Read the model definition and answer for the solid it produces. Units are mm, in the model's axes. A direction names the side the tool comes from. Give positions to 0.01 mm unless a question says otherwise; leave off trailing zeros. Order: outer loops, then holes, each group sorted by start corner. A loop starts at its lowest first (then second) coordinate and runs counter-clockwise, first axis right, second up.
Solid Edge part; units mm, degrees
sketch "Sketch1" plane through (0, 0, 0) normal (0, 0, 1) x (1, 0, 0)
  line L0 (0, -15) -> (120, -15)
  line L1 (0, 15) -> (120, 15)
  arc A0 (120, 15) -> (120, -15) centre (120, 0) cw
  arc A1 (0, -15) -> (0, 15) centre (0, 0) cw
extrude "Protrusion1" add sketch "Sketch1" against normal blind 6
sketch "Sketch2" plane through (0, 0, 0) normal (0, 0, 1) x (1, 0, 0)
  circle A0 centre (0, 0) radius 8
  circle A1 centre (120, 0) radius 8
extrude "VaciadoExtruido_1" cut sketch "Sketch2" against normal blind 5
sketch "Sketch3" plane through (0, 0, -5) normal (0, 0, 1) x (1, 0, 0)
  circle A0 centre (0, 0) radius 4.5
  circle A1 centre (120, 0) radius 4.5
extrude "Cutout1" cut sketch "Sketch3" against normal through all
chamfer "Chaflán_1" distance 3 angle 45 4 edges at (60, -15, -6) (135, 0, -6) (60, 15, -6) (-15, 0, -6)
1) For a pull along Y with two mould halves and no side action, classify faces 3 (the face through (135, 0, -1)), 4 (the face through (123.4, -3.4, -5)), 5 (the face through (59, -13, -5)) as released by +Y, released by -Y, zero draft, split by the parting line, or undercut.
Final values:
face 3: split by the parting line
face 4: undercut
face 5: released by -Y
2) Given pin 1 (5 mm diameter, centred on x = 124, y = 3, fed in from +Z); pin 2 (1 mm diameter, centred on x = 104, z = -4, fed in from +Y); pin 3 (1 mm diameter, centred on x = 105.5, z = -5, fed in from +Y), each flat-ended and moving along its own axis, determine where each tip first touches the part or whether it passes through.
Final values:
pin 1: stops at z = -5
pin 2: stops at y = 14.5
pin 3: stops at y = 13.5
3) A tool of negligible diameter and unlimited length cuts with its end or side. For faces 1 (the face through (127.63, 2.4, -2.46)), 2 (the face through (-0.59, 4.46, -5.49)), from which of +Z, -Z, +X, -X, +Y, -Y can it reach the whole face along a straight path? Write none if from no direction.
Final values:
face 1: +Z
face 2: +Z, -Z
4) Consider L1, parallel to X at y = -6.5, z = -0.6; L2, parallel to X at y = 0.75, z = -1.85; L3, parallel to Y at x = 120, z = -1.35. Determine where each line is inside the solid, lowest interval first.
Final values:
L1: x = -13.52 to -4.66, 4.66 to 115.34, 124.66 to 133.52
L2: x = -14.98 to -7.96, 7.96 to 112.04, 127.96 to 134.98
L3: y = -15 to -8, 8 to 15
5) The part is cut by section A-A on y = 0. Determine the outline of the cut face in (x, z), and give its area (3 significant figures).
Final values:
outline: (-15, -3) - (-12, -6) - (-4.5, -6) - (-4.5, -5) - (-8, -5) - (-8, 0) - (-15, 0) - close; (4.5, -6) - (115.5, -6) - (115.5, -5) - (112, -5) - (112, 0) - (8, 0) - (8, -5) - (4.5, -5) - close; (124.5, -6) - (132, -6) - (135, -3) - (135, 0) - (128, 0) - (128, -5) - (124.5, -5) - close
area: 713 mm2
6) The part is cut by section C-C on x = 110.5. Determine the outline of the cut face in (y, z).
Final values:
outline: (-15, -3) - (-12, -6) - (12, -6) - (15, -3) - (15, 0) - (-15, 0) - close
7) The part is cut by section B-B on z = -1.3. Determine the outline of the cut face in (x, y), and give its area (3 significant figures).
Final values:
outline: (0, -15) - (120, -15) arc R15 ccw to (120, 15) - (0, 15) arc R15 ccw to start; hole circle Ø16 at (0, 0); hole circle Ø16 at (120, 0)
area: 3,900 mm2
